Design review of the part shown in the three views and the two pictorial views. Dimensions are in mm from the part's minimum x, y and z. A direction names the side the tool comes from. Coordinates: 2 decimals unless noted, no trailing zeros. Order: outer loops, then holes, each group sorted by start corner. A loop starts at its lowest first (then second) coordinate and runs counter-clockwise, first axis right, second up. Notation, with made-up numbers: (-5.75, 67.25) -> (52.25, 67.25) arc R13 ccw to (52.25, 92.25) -> close; hole circle Ø9 at (13.5, 25.5). An arc over 180 degrees is marked (long way). Write item = value, one per line. Start each with the question number.
1) Consider section D-D on z = 20. Give the boundary of the cut face in (x, y), and give its area (3 significant figures).
2) Wall thickness on probe 1 along Y at (x, z) = (26, 3.15); probe 2 along Z at (x, y) = (1.65, 35); probe 3 along X at (y, z) = (87, 1.3): over which ranges is each line inside the solid? List them lowest first. Write a range as [from, to].
3) Insertion check: pin 1 Ø6 at (x, y) = (39, 43) entering from +Z; pin 2 Ø5 at (x, y) = (44.5, 81.5) entering from -Z. Each pin has a flat end and moves straight along its axis. Give the tip position at first contact, or say it passes through.
4) Consider section B-B on z = 36. Give the boundary of the cut face in (x, y), and give its area (3 significant figures).
5) Machinability: for the marked faces 1 and 2, which of the approach directions +Z, -Z, +X, -X, +Y, -Y give a long, thin tool a straight path to every point of the face, cutting with its end or side? Answer none if there is none.
6) Consider section C-C on y = 87. Give the boundary of the cut face in (x, z), and give its area (3 significant figures).
7) Draft analysis for pull direction X (two halves, no side actions). For the marked faces 3, 4 and 5, state which applies: +X half, -X half, draft (parallel to the pull), parting line (faces both ways), or undercut.
8) Consider section A-A on x = 54. Give the boundary of the cut face in (y, z).
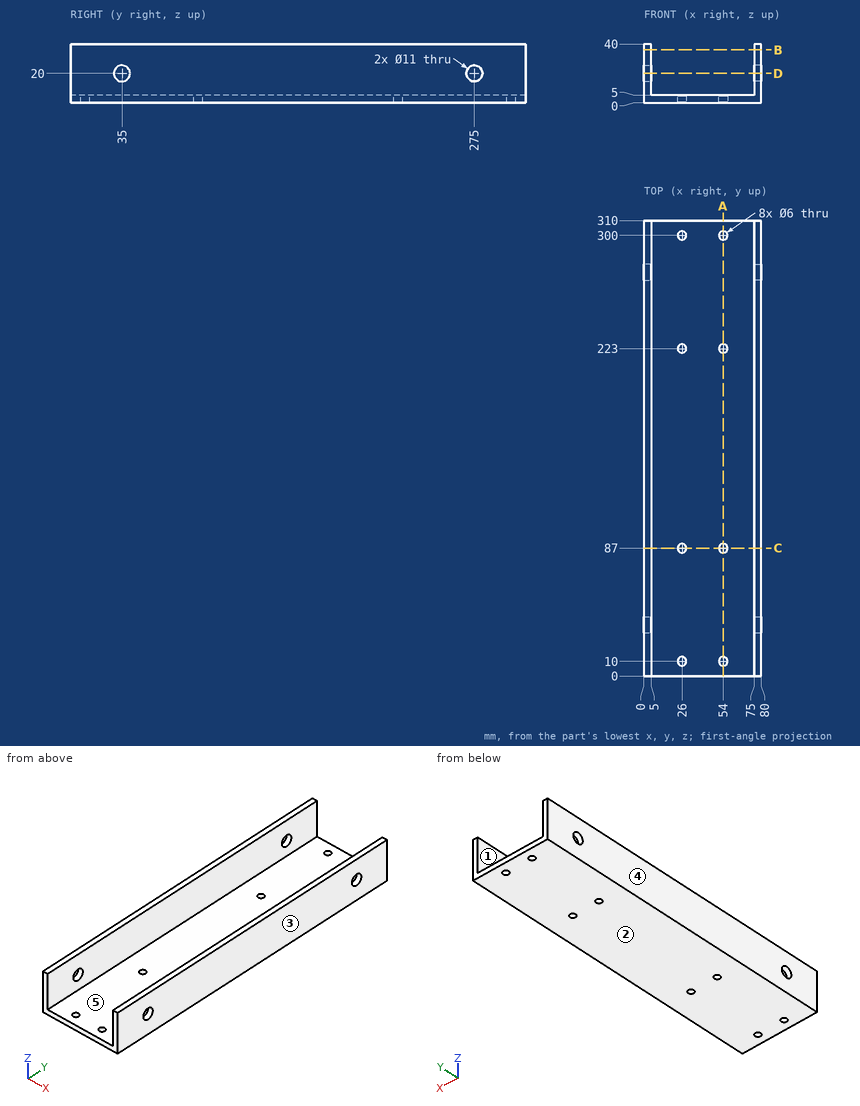
Answer sheet:
q1.outline = (0, 0) -> (5, 0) -> (5, 29.5) -> (0, 29.5) -> close; (0, 40.5) -> (5, 40.5) -> (5, 269.5) -> (0, 269.5) -> close; (0, 280.5) -> (5, 280.5) -> (5, 310) -> (0, 310) -> close; (75, 0) -> (80, 0) -> (80, 29.5) -> (75, 29.5) -> close; (75, 40.5) -> (80, 40.5) -> (80, 269.5) -> (75, 269.5) -> close; (75, 280.5) -> (80, 280.5) -> (80, 310) -> (75, 310) -> close
q1.area = 2,880 mm2
q2.probe_1 = [0, 7], [13, 84], [90, 220], [226, 297], [303, 310]
q2.probe_2 = [0, 14.5], [25.5, 40]
q2.probe_3 = [0, 23], [29, 51], [57, 80]
q3.pin_1 = 5
q3.pin_2 = 0
q4.outline = (0, 0) -> (5, 0) -> (5, 310) -> (0, 310) -> close; (75, 0) -> (80, 0) -> (80, 310) -> (75, 310) -> close
q4.area = 3,100 mm2
q5.face_1 = +Z, +Y, -Y
q5.face_2 = -Z, +X, -X, +Y, -Y
q6.outline = (0, 0) -> (23, 0) -> (23, 5) -> (5, 5) -> (5, 40) -> (0, 40) -> close; (29, 0) -> (51, 0) -> (51, 5) -> (29, 5) -> close; (57, 0) -> (80, 0) -> (80, 40) -> (75, 40) -> (75, 5) -> (57, 5) -> close
q6.area = 690 mm2
q7.face_3 = +X half
q7.face_4 = -X half
q7.face_5 = undercut
q8.outline = (0, 0) -> (7, 0) -> (7, 5) -> (0, 5) -> close; (13, 0) -> (84, 0) -> (84, 5) -> (13, 5) -> close; (90, 0) -> (220, 0) -> (220, 5) -> (90, 5) -> close; (226, 0) -> (297, 0) -> (297, 5) -> (226, 5) -> close; (303, 0) -> (310, 0) -> (310, 5) -> (303, 5) -> close
